The listing builds one solid part. Answer for the finished solid, in the listing's coordinates (mm). Face numbers are marked on the shaded views. A direction names the side the tool comes from. Coordinates: 2 decimals unless noted, no trailing zeros. Order: outer loops, then holes, each group sorted by start corner. A loop starts at its lowest first (then second) coordinate and runs counter-clockwise, first axis right, second up. Notation, with made-up numbers: M 40,16 L 71,16 A29 ccw 71,43 Z; hole C 47,-34 d10. An arc over 180 degrees is marked long. One line per item, written item: value. Start each with the question number.
Q1. Straight lines are drawn through the part: line 1 along Y through (x, z) = (0, 2.8); line 2 along Z through (x, y) = (7.5, 2); line 3 along X through (y, z) = (2.5, 3). For each, find the intervals that lie inside material, in ascending order. Write a range as [from, to].
Q2. The part is cut by section D-D on x = 16. Give the vertices of the cut face in (y, z).
Q3. The part is cut by section A-A on x = 0. Give the vertices of the cut face in (y, z).
Q4. Each of these flat-tipped pins is pushed along its axis until it touches: pin 1 Ø2.5 at (x, z) = (-3.5, 5) entering from +Y; pin 2 Ø1.5 at (x, y) = (-6.5, -9.5) entering from -Z; pin 3 Ø2 at (y, z) = (11.5, 5) entering from -X; pin 4 Ø1.5 at (y, z) = (15, 5) entering from +X. Where does it stop, or does it pass through?
Q5. The part is cut by section B-B on y = 0. Give the vertices of the cut face in (x, z).
Q6. Determine the mould class of the marked faces 1, 2, 3 and 4 for opening direction Y: pulls with the +Y half, pulls with the -Y half, needs draft (parallel to the pull), parting line crosses it, or undercut.
Q7. For the marked faces 5 and 6, determine the directions among +Z, -Z, +X, -X, +Y, -Y from which every point of the face is accessible in a straight line to the end or side of a thin tool.
Q8. The part is cut by section C-C on z = 2.5. Give the vertices of the cut face in (x, y), then the cut area to 3 significant figures.
Autodesk Inventor part; units mm, degrees
ref_plane "Arbeitsebene2" through (17, 0, 0) normal (1, 0, 0) x (0, 1, 0)
ref_plane "XZ Plane" through (0, 0, 0) normal (0, 1, 0) x (-1, 0, 0)
ref_plane "XY Plane" through (0, 0, 0) normal (0, 0, 1) x (1, 0, 0)
sketch "Skizze1" plane through (0, 0, 0) normal (0, 0, 1) x (1, 0, 0)
  circle A0 centre (0, 0) radius 20
  dimension "d0" = 40
extrude "Extrusion1" add sketch "Skizze1" along normal blind 1
sketch "Skizze2" plane through (0, 0, 1) normal (0, 0, 1) x (1, 0, 0)
  circle A0 centre (0, 0) radius 20
  circle A1 centre (0, 0) radius 17
  dimension "d3" = 34
extrude "Extrusion2" add sketch "Skizze2" along normal blind 10 contours A1
sketch "Skizze3" plane through (0, 0, 11) normal (0, 0, 1) x (1, 0, 0)
  circle A0 centre (0, 0) radius 17
  circle A1 centre (0, 0) radius 20
  dimension "d6" = 40
extrude "Extrusion3" add sketch "Skizze3" along normal blind 1 contours A0 | A1
sketch "Skizze6" plane through (0, 0, 12) normal (0, 0, 1) x (1, 0, 0)
  circle A0 centre (0, 0) radius 20
  circle A1 centre (0, 0) radius 5.1
  dimension "d16" = 10.2
extrude "Extrusion6" cut sketch "Skizze6" against normal through all contours A1
sketch "Skizze7" plane through (0, 0, 0) normal (0, 1, 0) x (-1, 0, 0)
  line L0 (17, 1) -> (17, 11)
  line L1 (-17, 1) -> (-17, 11)
  line L2 (20, 0) -> (-20, 0)
  line L3 (20, 0) -> (20, 1)
  line L4 (20, 1) -> (-20, 1)
  line L5 (-17, 1) -> (-17, 11)
  line L6 (20, 0) -> (-20, 0)
  line L7 (-20, 0) -> (-20, 6)
  line L8 (-20, 6) -> (20, 6)
  line L9 (20, 6) -> (20, 0)
  line L10 (20, 12) -> (-20, 12)
  point P0 (0, 0)
  dimension "d19" = 6
  dimension "d20" = 12
extrude "Extrusion7" cut sketch "Skizze7" along normal through all both and the other way through all keep common part
ref_plane "Arbeitsebene2" through (17, 0, 0) normal (1, 0, 0) x (0, 1, 0)
sketch "Skizze9" plane through (17, 0, 0) normal (1, 0, 0) x (0, 1, 0)
  line L0 (17, 6) -> (-17, 6)
  circle A0 centre (0, 6) radius 1
  point P0 (0, 0)
  point P1 (-1, 6)
  point P2 (1, 6)
  dimension "d24" = 2
extrude "Extrusion8" cut sketch "Skizze9" against normal blind 5 contours A0 L0 picked at (0.0402, 5.6691)
sketch "Skizze10" plane through (12, 1, 6) normal (0, 0, 1) x (1, 0, 0)
  circle A0 centre (-12, -1) radius 5.1
  line L0 (-19.6, 6.6) -> (-4.4, 6.6)
  line L1 (-4.4, 6.6) -> (-4.4, -8.6)
  line L2 (-4.4, -8.6) -> (-19.6, -8.6)
  line L3 (-19.6, -8.6) -> (-19.6, 6.6)
  line L4 (-19.6, 6.6) -> (-4.4, -8.6) construction
  line L5 (-4.4, 6.6) -> (-19.6, -8.6) construction
  dimension "d27" = 15.2
  dimension "d28" = 15.2
extrude "Extrusion9" cut sketch "Skizze10" against normal blind 2.2
equation "\"d19\" = 0.5 * d20"
equation "\"d28\" = d27"
properties part number "Motorstange_version2b"
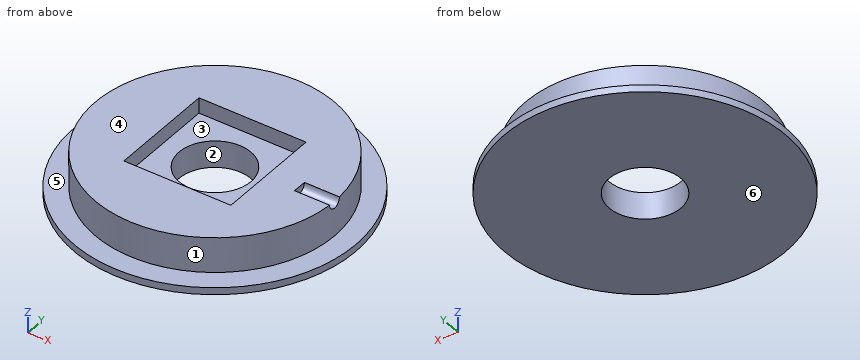
Output:
1. line 1: y = [-17, -5.1], [5.1, 17]
1. line 2: z = [0, 3.8]
1. line 3: x = [-16.82, -4.45], [4.45, 16.82]
2. outline: M -12,0 L 12,0 L 12,1 L 5.74,1 L 5.74,6 L 1,6 A1 cw -1,6 L -5.74,6 L -5.74,1 L -12,1 Z
3. outline: M -20,0 L -5.1,0 L -5.1,3.8 L -7.6,3.8 L -7.6,6 L -17,6 L -17,1 L -20,1 Z; M 5.1,0 L 20,0 L 20,1 L 17,1 L 17,6 L 7.6,6 L 7.6,3.8 L 5.1,3.8 Z
4. pin 1: stops at y = 16.85
4. pin 2: stops at z = 0
4. pin 3: stops at x = -13.37
4. pin 4: stops at x = 9.27
5. outline: M -20,0 L -5.1,0 L -5.1,3.8 L -7.6,3.8 L -7.6,6 L -17,6 L -17,1 L -20,1 Z; M 5.1,0 L 20,0 L 20,1 L 17,1 L 17,5 L 12,5 L 12,6 L 7.6,6 L 7.6,3.8 L 5.1,3.8 Z
6. face 1: parting line crosses it
6. face 2: undercut
6. face 3: undercut
6. face 4: needs draft
7. face 5: +Z
7. face 6: -Z, +X, -X, +Y, -Y
8. outline: C 0,0 d34; hole C 0,0 d10.2
8. area: 826 mm^2
